Autodesk Inventor part; units mm, degrees
ref_plane "YZ Plane" through (0, 0, 0) normal (1, 0, 0) x (0, 1, 0)
ref_plane "XZ Plane" through (0, 0, 0) normal (0, 1, 0) x (-1, 0, 0)
ref_plane "XY Plane" through (0, 0, 0) normal (0, 0, 1) x (1, 0, 0)
sketch "Sketch1" plane through (0, 0, 0) normal (0, 0, 1) x (1, 0, 0)
  circle A0 centre (76.6657, 1.1203) radius 3
  line L0 (88.1657, -4.2797) -> (97.1657, -4.2797)
  line L1 (97.1657, -4.2797) -> (97.1657, 4.1203)
  line L2 (97.1657, 4.1203) -> (88.1657, 4.1203)
  line L3 (124.4657, -12.1297) -> (124.4657, 14.6703)
  line L4 (88.1657, 4.1203) -> (88.1657, -4.2797)
  line L5 (56.0657, -2.0797) -> (56.0657, 5.8203)
  line L6 (33.6679, 7.1494) -> (33.6679, -2.7506)
  line L7 (32.8657, 14.6703) -> (32.8657, -12.1297)
  line L8 (31.4657, -2.0797) -> (56.0657, -2.0797)
  line L9 (56.0657, 5.8203) -> (31.4657, 5.8203)
  line L10 (124.4657, 14.6703) -> (-59.7343, 14.6703)
  line L11 (-59.7343, -5.3797) -> (124.4657, -5.3797)
  line L12 (-59.7343, -12.1297) -> (124.4657, -12.1297)
  line L13 (31.4657, 5.8203) -> (31.4657, -2.0797)
  line L14 (-59.7343, 14.6703) -> (-59.7343, -12.1297)
  line L15 (6.6657, -2.0797) -> (6.6657, 5.8203)
  line L16 (-17.9343, -2.0797) -> (6.6657, -2.0797)
  line L17 (-17.9343, 5.8203) -> (-17.9343, -2.0797)
  line L18 (6.6657, 5.8203) -> (-17.9343, 5.8203)
  line L19 (7.6657, 6.8203) -> (7.6657, -3.0797)
  line L20 (7.6657, -3.0797) -> (-18.9343, -3.0797)
  line L21 (-18.9343, -3.0797) -> (-18.9343, 6.8203)
  line L22 (-18.9343, 6.8203) -> (7.6657, 6.8203)
  line L23 (57.0657, 6.8203) -> (57.0657, -3.0797)
  line L24 (57.0657, -3.0797) -> (30.4657, -3.0797)
  line L25 (30.4657, -3.0797) -> (30.4657, 6.8203)
  line L26 (30.4657, 6.8203) -> (57.0657, 6.8203)
  circle A1 centre (76.6657, 1.1203) radius 4
  line L27 (98.1657, 5.1203) -> (98.1657, -5.2797)
  line L28 (98.1657, -5.2797) -> (87.1657, -5.2797)
  line L29 (87.1657, -5.2797) -> (87.1657, 5.1203)
  line L30 (87.1657, 5.1203) -> (98.1657, 5.1203)
  point P0 (0, 0)
  point P1 (0, 0)
  dimension "d1" = 6.75
  dimension "d2" = 7.9
  dimension "d3" = 24.6
  dimension "d4" = 3.3
  dimension "d5" = 3.3
  dimension "d6" = 24.6
  dimension "d7" = 7.9
  dimension "d8" = 24.8
  dimension "d10" = 6
  dimension "d11" = 6.5
  dimension "d12" = 20.6
  dimension "d13" = 9
  dimension "d14" = 1.1
  dimension "d15" = 8.4
  dimension "d17" = 1
  dimension "d18" = 1
  dimension "d19" = 1
  dimension "d20" = 1
  dimension "d27" = 11.5
  dimension "d30" = 26.8
  dimension "d32" = 41.8
  dimension "d33" = 184.2
extrude "Extrusion1" add sketch "Sketch1" along normal blind 1.9 contours L12 L7 L11 L3 | L11 L7 L24 L23 L26 L10 L3 | L12 L14 L11 L7 | L11 L14 L10 L7 L26 L25 L24
equation "\"BendRadius\" = Thickness"
equation "\"BendReliefWidth\" = Thickness"
equation "\"BendReliefDepth\" = 0.5 * Thickness"
equation "\"CornerReliefSize\" = 4 * Thickness"
equation "\"MinimumRemnant\" = 2 * Thickness"
equation "\"TransitionRadius\" = BendRadius"
equation "\"JacobiRadiusSize\" = BendRadius"
equation "\"GapSize\" = Thickness"
properties part number "panel 2"
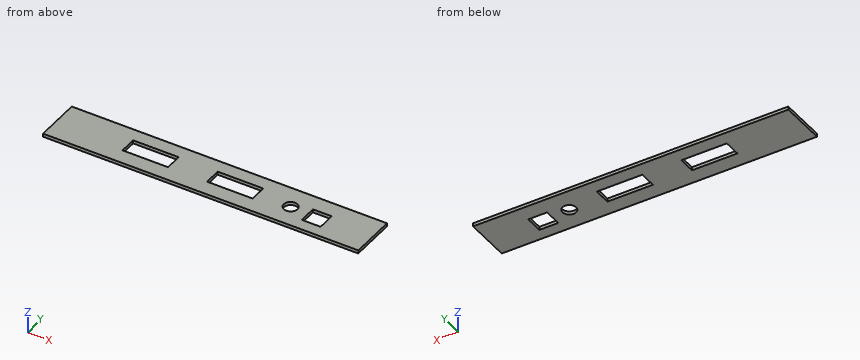
Here's how the part is built. I have some questions about the finished solid (model axes, mm). Give positions to 0.01 mm unless a question says otherwise; leave off trailing zeros. Loops run counter-clockwise (first coordinate to the right, second up) from the corner with the lowest first, then second, coordinate; pieces in that order, holes last. Notation, with made-up numbers: M 80,-38.75 L 120,-38.75 A10 cw 120,-27.75 Z; hole C 11.5,-36 d4. An arc over 180 degrees is marked long. Use one line per item in the form item = value. Start each with the question number.
Q1. I need wall thicknesses on line 1 along X through (y, z) = (5.75, 0.95); line 2 along Y through (x, z) = (-16, 0.55); line 3 along Y through (x, z) = (87.5, 1.4). Which ranges of each line are inside material? Lowest first, please.
Q2. If we section it at C-C (z = 1.6): Write out the boundary of the cut face in (x, y), then the cut area to 3 significant figures.
Q3. If we section it at A-A (x = -1): Write out the boundary of the cut face in (y, z), then the cut area to 3 significant figures.
Q4. If we section it at B-B (y = 3): Write out the boundary of the cut face in (x, z).
Taken from the geometry:
q1.line_1 = -59.73 to -18.93, 7.67 to 30.47, 57.07 to 124.47
q1.line_2 = -12.13 to -3.08, 6.82 to 14.67
q1.line_3 = -12.13 to -5.28, 5.12 to 14.67
q2.outline = M -59.73,-12.13 L 124.47,-12.13 L 124.47,14.67 L -59.73,14.67 Z; hole M -18.93,-3.08 L 7.67,-3.08 L 7.67,6.82 L -18.93,6.82 Z; hole M 30.47,-3.08 L 57.07,-3.08 L 57.07,6.82 L 30.47,6.82 Z; hole C 76.67,1.12 d8; hole M 87.17,-5.28 L 98.17,-5.28 L 98.17,5.12 L 87.17,5.12 Z
q2.area = 4,250 mm^2
q3.outline = M -12.13,0 L -3.08,0 L -3.08,1.9 L -12.13,1.9 Z; M 6.82,0 L 14.67,0 L 14.67,1.9 L 6.82,1.9 Z
q3.area = 32.1 mm^2
q4.outline = M -59.73,0 L -18.93,0 L -18.93,1.9 L -59.73,1.9 Z; M 7.67,0 L 30.47,0 L 30.47,1.9 L 7.67,1.9 Z; M 57.07,0 L 73.13,0 L 73.13,1.9 L 57.07,1.9 Z; M 80.2,0 L 87.17,0 L 87.17,1.9 L 80.2,1.9 Z; M 98.17,0 L 124.47,0 L 124.47,1.9 L 98.17,1.9 Z
